```python
from build123d import *

# Parameters (mm, degrees)
CROQUIS1_W              = 41
CROQUIS1_H              = 41
SALIENTE_EXTRUIR1_DEPTH = 15.5
CHAFL_N1_SIZE           = 5
REDONDEO1_R             = 3
CROQUIS2_W              = 41.1
CROQUIS2_H              = 41.1
SALIENTE_EXTRUIR2_DEPTH = 8
CHAFL_N2_SIZE           = 3
SALIENTE_EXTRUIR3_DEPTH = 9
CROQUIS4_R              = 11
SALIENTE_EXTRUIR4_DEPTH = 2
CROQUIS5_R              = 1.190625
CORTAR_EXTRUIR1_DEPTH   = 3.175
CHAFL_N3_SIZE           = 0.1
CROQUIS6_R              = 4.7625
CROQUIS6_R_2            = 3.175
CORTAR_EXTRUIR2_DEPTH   = 3
C_PULA1_FACE_RADIUS     = 3.175
C_PULA1_HEIGHT          = 3
C_PULA2_FACE_RADIUS     = 3.175
C_PULA2_HEIGHT          = 3
C_PULA3_FACE_RADIUS     = 3.175
C_PULA3_HEIGHT          = 3
C_PULA4_FACE_RADIUS     = 3.175
C_PULA4_HEIGHT          = 3
CROQUIS7_R              = 4.5
CORTAR_EXTRUIR3_DEPTH   = 3
SALIENTE_EXTRUIR5_DEPTH = 24.43125
CORTAR_EXTRUIR4_DEPTH   = 20.5


with BuildPart() as part:
    # Croquis1 → Saliente-Extruir1 (new body, symmetric)
    with BuildSketch(Plane(origin=(0, 0, 0), x_dir=(1, 0, 0), z_dir=(0, 1, 0))):
        Rectangle(CROQUIS1_W, CROQUIS1_H)
    extrude(amount=SALIENTE_EXTRUIR1_DEPTH, both=True)

    # Chaflán1
    chafl_n1_edges = [part.edges().sort_by_distance(p)[0] for p in [
        (20.5, 0, 20.5),
        (-20.5, 0, 20.5),
        (-20.5, 0, -20.5),
        (20.5, 0, -20.5),
    ]]
    chamfer(chafl_n1_edges, length=CHAFL_N1_SIZE)

    # Redondeo1
    redondeo1_edges = [part.edges().sort_by_distance(p)[0] for p in [
        (15.5, 0, 20.5),
        (-15.5, 0, 20.5),
        (-20.5, 0, -15.5),
        (-20.5, 0, 15.5),
        (15.5, 0, -20.5),
        (-15.5, 0, -20.5),
        (20.5, 0, 15.5),
        (20.5, 0, -15.5),
    ]]
    fillet(redondeo1_edges, radius=REDONDEO1_R)

    # Croquis2 → Saliente-Extruir2 (add)
    with BuildSketch(Plane(origin=(0, 15.5, 0), x_dir=(1, 0, 0), z_dir=(0, 1, 0))):
        Rectangle(CROQUIS2_W, CROQUIS2_H)
    extrude(amount=SALIENTE_EXTRUIR2_DEPTH)

    # Chaflán2
    chafl_n2_edges = [part.edges().sort_by_distance(p)[0] for p in [
        (20.55, 19.5, 20.55),
        (20.55, 19.5, -20.55),
        (-20.55, 19.5, -20.55),
        (-20.55, 19.5, 20.55),
    ]]
    chamfer(chafl_n2_edges, length=CHAFL_N2_SIZE)

    # Croquis3 → Saliente-Extruir3 (add)
    with BuildSketch(Plane.XZ.offset(15.5)):
        Polygon((17.55, 20.55), (-17.55, 20.55), (-20.55, 17.55), (-20.55, -17.55), (-17.55, -20.55), (17.55, -20.55), (20.55, -17.55), (20.55, 17.55), align=None)
    extrude(amount=SALIENTE_EXTRUIR3_DEPTH)

    # Croquis4 → Saliente-Extruir4 (add)
    with BuildSketch(Plane(origin=(0, 23.5, 0), x_dir=(1, 0, 0), z_dir=(0, 1, 0))):
        Circle(CROQUIS4_R)
    extrude(amount=SALIENTE_EXTRUIR4_DEPTH)

    # Croquis5 → Cortar-Extruir1 (cut)
    with BuildSketch(Plane(origin=(0, 23.5, 0), x_dir=(1, 0, 0), z_dir=(0, 1, 0))):
        with Locations((-15.5, 15.5)):
            Circle(CROQUIS5_R)
        with Locations((15.5, 15.5)):
            Circle(CROQUIS5_R)
        with Locations((15.5, -15.5)):
            Circle(CROQUIS5_R)
        with Locations((-15.5, -15.5)):
            Circle(CROQUIS5_R)
    extrude(amount=-CORTAR_EXTRUIR1_DEPTH, mode=Mode.SUBTRACT)

    # Chaflán3
    chafl_n3_edges = [part.edges().sort_by_distance(p)[0] for p in [
        (-16.690625, 23.5, -15.5),
        (14.309375, 23.5, -15.5),
        (14.309375, 23.5, 15.5),
        (-16.690625, 23.5, 15.5),
    ]]
    chamfer(chafl_n3_edges, length=CHAFL_N3_SIZE)

    # Croquis6 → Cortar-Extruir2 (cut)
    with BuildSketch(Plane.XZ.offset(24.5)):
        Circle(CROQUIS6_R)
        with Locations((-15.5, 15.5)):
            Circle(CROQUIS6_R_2)
        with Locations((15.5, 15.5)):
            Circle(CROQUIS6_R_2)
        with Locations((15.5, -15.5)):
            Circle(CROQUIS6_R_2)
        with Locations((-15.5, -15.5)):
            Circle(CROQUIS6_R_2)
    extrude(amount=-CORTAR_EXTRUIR2_DEPTH, mode=Mode.SUBTRACT)

    # Cúpula1: a dome of height H over a round flat face of radius A is a cap of a sphere of radius (A * A + H * H) / (2 * H)
    c_pula1_r = (C_PULA1_FACE_RADIUS * C_PULA1_FACE_RADIUS + C_PULA1_HEIGHT * C_PULA1_HEIGHT) / (2 * C_PULA1_HEIGHT)
    c_pula1_base = Plane((15.5, -21.5, 15.5), z_dir=(0, -1, 0))
    with Locations(c_pula1_base.offset(C_PULA1_HEIGHT - c_pula1_r)):
        c_pula1_ball = Sphere(c_pula1_r, mode=Mode.PRIVATE)
    add(split(c_pula1_ball, bisect_by=c_pula1_base, keep=Keep.TOP, mode=Mode.PRIVATE))

    # Cúpula2: a dome of height H over a round flat face of radius A is a cap of a sphere of radius (A * A + H * H) / (2 * H)
    c_pula2_r = (C_PULA2_FACE_RADIUS * C_PULA2_FACE_RADIUS + C_PULA2_HEIGHT * C_PULA2_HEIGHT) / (2 * C_PULA2_HEIGHT)
    c_pula2_base = Plane((-15.5, -21.5, 15.5), z_dir=(0, -1, 0))
    with Locations(c_pula2_base.offset(C_PULA2_HEIGHT - c_pula2_r)):
        c_pula2_ball = Sphere(c_pula2_r, mode=Mode.PRIVATE)
    add(split(c_pula2_ball, bisect_by=c_pula2_base, keep=Keep.TOP, mode=Mode.PRIVATE))

    # Cúpula3: a dome of height H over a round flat face of radius A is a cap of a sphere of radius (A * A + H * H) / (2 * H)
    c_pula3_r = (C_PULA3_FACE_RADIUS * C_PULA3_FACE_RADIUS + C_PULA3_HEIGHT * C_PULA3_HEIGHT) / (2 * C_PULA3_HEIGHT)
    c_pula3_base = Plane((15.5, -21.5, -15.5), z_dir=(0, -1, 0))
    with Locations(c_pula3_base.offset(C_PULA3_HEIGHT - c_pula3_r)):
        c_pula3_ball = Sphere(c_pula3_r, mode=Mode.PRIVATE)
    add(split(c_pula3_ball, bisect_by=c_pula3_base, keep=Keep.TOP, mode=Mode.PRIVATE))

    # Cúpula4: a dome of height H over a round flat face of radius A is a cap of a sphere of radius (A * A + H * H) / (2 * H)
    c_pula4_r = (C_PULA4_FACE_RADIUS * C_PULA4_FACE_RADIUS + C_PULA4_HEIGHT * C_PULA4_HEIGHT) / (2 * C_PULA4_HEIGHT)
    c_pula4_base = Plane((-15.5, -21.5, -15.5), z_dir=(0, -1, 0))
    with Locations(c_pula4_base.offset(C_PULA4_HEIGHT - c_pula4_r)):
        c_pula4_ball = Sphere(c_pula4_r, mode=Mode.PRIVATE)
    add(split(c_pula4_ball, bisect_by=c_pula4_base, keep=Keep.TOP, mode=Mode.PRIVATE))

    # Croquis7 → Cortar-Extruir3 (cut)
    with BuildSketch(Plane(origin=(0, 25.5, 0), x_dir=(1, 0, 0), z_dir=(0, 1, 0))):
        Circle(CROQUIS7_R)
    extrude(amount=-CORTAR_EXTRUIR3_DEPTH, mode=Mode.SUBTRACT)

    # Croquis8 → Saliente-Extruir5 (add)
    with BuildSketch(Plane(origin=(0, 22.5, 0), x_dir=(1, 0, 0), z_dir=(0, 1, 0))):
        with BuildLine():
            ThreePointArc((2.5, 0), (0.612372436, 2.423839929), (-2.2, 1.187434209))
            Line((-2.2, 1.187434209), (-2.2, -1.187434209))
            ThreePointArc((-2.2, -1.187434209), (0.612372436, -2.423839929), (2.5, 0))
        make_face()
        with BuildLine():
            Line((-2.2, -1.187434209), (-2.2, 1.187434209))
            ThreePointArc((-2.2, 1.187434209), (-2.5, 0), (-2.2, -1.187434209))
        make_face()
    extrude(amount=SALIENTE_EXTRUIR5_DEPTH)

    # Croquis9 → Cortar-Extruir4 (cut)
    with BuildSketch(Plane(origin=(0, 46.93125, 0), x_dir=(1, 0, 0), z_dir=(0, 1, 0))):
        with BuildLine():
            Line((-2.2, -1.187434209), (-2.2, 1.187434209))
            ThreePointArc((-2.2, 1.187434209), (-2.5, 0), (-2.2, -1.187434209))
        make_face()
    extrude(amount=-CORTAR_EXTRUIR4_DEPTH, mode=Mode.SUBTRACT)


solid = part.part
```
The model under review builds one solid part; all positions refer to its coordinate system, in mm. A direction names the side the tool comes from. Round coordinates to 2 decimals unless told otherwise and drop trailing zeros. Order: outer loops, then holes, each group sorted by start corner. A loop starts at its lowest first (then second) coordinate and runs counter-clockwise, first axis right, second up. Notation, with made-up numbers: (81.5, 14) -> (86.5, 14) arc R23 cw to (86.5, 30) -> close; hole circle Ø10 at (38, 67.5). An arc over 180 degrees is marked (long way). One line per item, written item: value. Start each with the question number.
Q1. Wall thickness on line 1 (X direction, y = 22.4, z = -15.5); line 2 (Z direction, x = 0, y = 23.6); line 3 (X direction, y = -22.75, z = 15.5) (3 decimals): over which ranges is each line inside the solid? List them lowest first.
Q2. Take a section at D-D (x = 8). Write out the cut boundary in (y, z), and give its area (3 significant figures).
Q3. Take a section at A-A (x = 0). Write out the cut boundary in (y, z), and give its area (3 significant figures).
Q4. Machinability: for faces 5 (the face through (-20.55, -20, 0)), 6 (the face through (15.39, -0.22, -20.28)), 7 (the face through (18.2, 15.5, 18.2)), 8 (the face through (-18, 0, 18)), 9 (the face through (-16, 20.325, -16)), which of the approach directions +Z, -Z, +X, -X, +Y, -Y give a long, thin tool a straight path to every point of the face, cutting with its end or side? Answer none if there is none.
Q5. Take a section at B-B (y = 14). Write out the cut boundary in (x, z), and give its area (3 significant figures).
Q6. Clearance check with flat-ended pins moving along their axes: pin 1 Ø4 at (y, z) = (35.5, -4) entering from -X; pin 2 Ø5 at (x, z) = (15.5, -15.5) entering from +Y; pin 3 Ø8.5 at (y, z) = (-2, -3.5) entering from -X. State where each tip first meets the part, or that it passes through.
Q7. Mouldability with a two-part tool opening along Z and no side actions: class faces 1 (the face through (-15.421, -0.217, -20.265)), 2 (the face through (-19, -19.9, 19.1)), 3 (the face through (-3.78, -23.02, -2.9)), 4 (the face through (20.5, 0, 0)) as released by +Z, released by -Z, zero draft, split by the parting line, or undercut.
Reported:
1. line 1: x = -20.55 to -16.69, -14.31 to 14.31, 16.69 to 20.55
1. line 2: z = -11 to -4.5, -2.5 to 2.5, 4.5 to 11
1. line 3: x = -20.55 to -18.675, -18.34 to -12.66, -12.325 to 12.325, 12.66 to 18.34, 18.675 to 20.55
2. outline: (-24.5, -20.55) -> (-15.5, -20.55) -> (-15.5, -20.5) -> (15.5, -20.5) -> (15.5, -20.55) -> (23.5, -20.55) -> (23.5, -7.55) -> (25.5, -7.55) -> (25.5, 7.55) -> (23.5, 7.55) -> (23.5, 20.55) -> (15.5, 20.55) -> (15.5, 20.5) -> (-15.5, 20.5) -> (-15.5, 20.55) -> (-24.5, 20.55) -> close
2. area: 2,000 mm2
3. outline: (-24.5, -20.55) -> (-15.5, -20.55) -> (-15.5, -20.5) -> (15.5, -20.5) -> (15.5, -20.55) -> (23.5, -20.55) -> (23.5, -11) -> (25.5, -11) -> (25.5, -4.5) -> (22.5, -4.5) -> (22.5, -2.5) -> (46.93, -2.5) -> (46.93, 2.5) -> (22.5, 2.5) -> (22.5, 4.5) -> (25.5, 4.5) -> (25.5, 11) -> (23.5, 11) -> (23.5, 20.55) -> (15.5, 20.55) -> (15.5, 20.5) -> (-15.5, 20.5) -> (-15.5, 20.55) -> (-24.5, 20.55) -> (-24.5, 4.76) -> (-21.5, 4.76) -> (-21.5, -4.76) -> (-24.5, -4.76) -> close
3. area: 2,080 mm2
4. face 5: +Z, -Z, -X, +Y, -Y
4. face 6: -Z, +X
4. face 7: none
4. face 8: +Z, -X
4. face 9: +Y
5. outline: (-20.5, -14.26) arc R3 ccw to (-19.62, -16.38) -> (-16.38, -19.62) arc R3 ccw to (-14.26, -20.5) -> (14.26, -20.5) arc R3 ccw to (16.38, -19.62) -> (19.62, -16.38) arc R3 ccw to (20.5, -14.26) -> (20.5, 14.26) arc R3 ccw to (19.62, 16.38) -> (16.38, 19.62) arc R3 ccw to (14.26, 20.5) -> (-14.26, 20.5) arc R3 ccw to (-16.38, 19.62) -> (-19.62, 16.38) arc R3 ccw to (-20.5, 14.26) -> close
5. area: 1,630 mm2
6. pin 1: stops at x = -1.5
6. pin 2: stops at y = 23.5
6. pin 3: stops at x = -20.5
7. face 1: released by -Z
7. face 2: released by +Z
7. face 3: undercut
7. face 4: zero draft
